Source: CAD feature listing. Evaluate the final solid. Frame: model axes, mm. A direction names the side the tool comes from. Round coordinates to 2 decimals unless told otherwise and drop trailing zeros. Order: outer loops, then holes, each group sorted by start corner. A loop starts at its lowest first (then second) coordinate and runs counter-clockwise, first axis right, second up. Notation, with made-up numbers: (-13, -24) - (1, -24) arc R17 ccw to (1, 2) - close; hole circle Ø8 at (-31.75, 12.25). An arc over 180 degrees is marked (long way). Return JSON: item names as keys, results as strings. Group by question number.
1) Section C-C, the plane x = 1. Return loops of the section in (y, z), plus the area to 3 significant figures.
2) Ray query, line 1 (Y direction, x = -16.5, z = 52.5); line 2 (Z direction, x = 4, y = -27); line 3 (Y direction, x = 34, z = 57.5). Return the intervals inside material, ascending. Write a range as from..to.
3) Section A-A, the plane z = 93. Return loops of the section in (x, y), plus the area to 3 significant figures.
4) Section D-D, the plane y = -35. Return loops of the section in (x, z).
5) Access query for faces 1 (the flat face through (-33.936, 19.961, 64.033)), 2 (the flat face through (0, -41.91, 50)), 3 (the flat face through (34, -20, 19.05)). Directions: +Z, -Z, +X, -X, +Y, -Y. A direction counts if a zero-diameter tool reaches every point of the face in a straight line with its end or side. Return the directions, or none.
6) Mould query, pull axis Z, two halves, no side actions, for faces 4 (the flat face through (0, -40, 19.05)), 5 (the flat face through (36, 19, 101.6)), 6 (the flat face through (33.936, -19.961, 64.033)). Classes: pulls with the +Z half, pulls with the -Z half, needs draft (parallel to the pull), parting line crosses it, or undercut.
7) Contact query for flat-ended pins moving along their axis: P1, Ø10, axis at y = -26, z = 28.5, coming from the +X side; P2, Ø8, axis at x = -37.5, z = 67.5, coming from the +Y side; P3, Ø1.3, axis at x = -3.5, y = 40, coming from the -Z side. Output: stop coordinate, or through.
```python
from build123d import *

# Parameters (mm, degrees)
F1_DEPTH = 101.6
F3_DEPTH = 76.2
F5_DEPTH = 19.05


with BuildPart() as f1:
    # F0 (on Top) → F1 (new body)
    with BuildSketch(Plane.XY):
        Polygon((-24.19675, -41.91), (24.19675, -41.91), (48.3935, 0), (24.19675, 41.91), (-24.19675, 41.91), (-48.3935, 0), align=None)
    extrude(amount=F1_DEPTH)

    # F2 (on face) → F3 (cut)
    with BuildSketch(Plane.XY.offset(101.6)):
        Polygon((-22.73028, -39.37), (22.73028, -39.37), (45.46056, 0), (22.73028, 39.37), (-22.73028, 39.37), (-45.46056, 0), align=None)
    extrude(amount=-F3_DEPTH, mode=Mode.SUBTRACT)

    # F4 (on face) → F5 (cut)
    with BuildSketch(Plane(origin=(0, 0, 0), x_dir=(1, 0, 0), z_dir=(0, 0, -1))):
        Polygon((-7.62, 37.510591), (0, 37.510591), (0, 41.91), (-5.08, 41.91), align=None)
        Polygon((7.62, 37.510591), (5.08, 41.91), (0, 41.91), (0, 37.510591), align=None)
        Polygon((32.485125, 18.755295), (36.295125, 20.955), (33.755125, 25.354409), (28.675125, 25.354409), align=None)
        Polygon((36.295125, 12.156182), (38.835125, 16.555591), (36.295125, 20.955), (32.485125, 18.755295), align=None)
        Polygon((36.295125, -20.955), (38.835125, -16.555591), (36.295125, -12.156182), (32.485125, -18.755295), align=None)
        Polygon((33.755125, -25.354409), (36.295125, -20.955), (32.485125, -18.755295), (28.675125, -25.354409), align=None)
        Polygon((7.62, -37.510591), (0, -37.510591), (0, -41.91), (5.08, -41.91), align=None)
        Polygon((0, -41.91), (0, -37.510591), (-7.62, -37.510591), (-5.08, -41.91), align=None)
        Polygon((-28.675125, -25.354409), (-32.485125, -18.755295), (-36.295125, -20.955), (-33.755125, -25.354409), align=None)
        Polygon((-36.295125, -20.955), (-32.485125, -18.755295), (-36.295125, -12.156182), (-38.835125, -16.555591), align=None)
        Polygon((-36.295125, 20.955), (-32.485125, 18.755295), (-28.675125, 25.354409), (-33.755125, 25.354409), align=None)
        Polygon((-36.295125, 12.156182), (-32.485125, 18.755295), (-36.295125, 20.955), (-38.835125, 16.555591), align=None)
    extrude(amount=-F5_DEPTH, mode=Mode.SUBTRACT)


solid = f1.part
```
Geometry check:
{
 "1": {"outline": "(-41.91, 19.05) - (-37.51, 19.05) - (-37.51, 0) - (37.51, 0) - (37.51, 19.05) - (41.91, 19.05) - (41.91, 101.6) - (39.37, 101.6) - (39.37, 25.4) - (-39.37, 25.4) - (-39.37, 101.6) - (-41.91, 101.6) - close", "area": "2,350 mm2"},
 "2": {"line 1": "-41.91..-39.37, 39.37..41.91", "line 2": "0..25.4", "line 3": "-24.93..-19.85, 19.85..24.93"},
 "3": {"outline": "(-48.39, 0) - (-24.2, -41.91) - (24.2, -41.91) - (48.39, 0) - (24.2, 41.91) - (-24.2, 41.91) - close; hole (-45.46, 0) - (-22.73, -39.37) - (22.73, -39.37) - (45.46, 0) - (22.73, 39.37) - (-22.73, 39.37) - close", "area": "715 mm2"},
 "4": {"outline": "(-28.19, 0) - (28.19, 0) - (28.19, 101.6) - (25.25, 101.6) - (25.25, 25.4) - (-25.25, 25.4) - (-25.25, 101.6) - (-28.19, 101.6) - close"},
 "5": {"face 1": "+Z", "face 2": "+Z, -Z, +X, -X, -Y", "face 3": "-Z"},
 "6": {"face 4": "pulls with the -Z half", "face 5": "pulls with the +Z half", "face 6": "needs draft"},
 "7": {"P1": "x = 36.27", "P2": "y = 25.8", "P3": "z = 19.05"}
}
